The listing builds one solid part. Answer for the finished solid, in the listing's coordinates (mm). Coordinates: 2 decimals unless noted, no trailing zeros. Write each loop counter-clockwise with the first axis right and the second up, starting at its lowest first coordinate (ties: lowest second). Pieces come first, ordered by that corner, then holes.
from build123d import *

# Parameters (mm, degrees)
SKETCH_1_R          = 1.525
EXTRUDE_1_DEPTH     = 3
FILLET_1_R          = 4
CUT_EXTRUDE_1_DEPTH = 10
FILLET_2_R          = 2
SKETCH_4_R          = 2.5
CUT_EXTRUDE_2_DEPTH = 10
FILLET_3_R          = 2


with BuildPart() as part:
    # 草图1 → 凸台-拉伸1 (new body)
    with BuildSketch(Plane.XY):
        with BuildLine():
            Line((75, -15), (75, 15))
            Line((75, 15), (42.759879905, 24.346070366))
            ThreePointArc((42.759879905, 24.346070366), (42.136261187, 24.480044275), (41.5, 24.525))
            Line((41.5, 24.525), (-41.5, 24.525))
            ThreePointArc((-41.5, 24.525), (-42.136261187, 24.480044275), (-42.759879905, 24.346070366))
            Line((-42.759879905, 24.346070366), (-75, 15))
            Line((-75, 15), (-75, -15))
            Line((-75, -15), (-42.759879905, -24.346070366))
            ThreePointArc((-42.759879905, -24.346070366), (-42.136261187, -24.480044275), (-41.5, -24.525))
            Line((-41.5, -24.525), (41.5, -24.525))
            ThreePointArc((41.5, -24.525), (42.136261187, -24.480044275), (42.759879905, -24.346070366))
            Line((42.759879905, -24.346070366), (75, -15))
        make_face()
        with Locations((-71, -10)):
            Circle(SKETCH_1_R, mode=Mode.SUBTRACT)
        with Locations((71, -10)):
            Circle(SKETCH_1_R, mode=Mode.SUBTRACT)
        with Locations((-71, 10)):
            Circle(SKETCH_1_R, mode=Mode.SUBTRACT)
        with Locations((71, 10)):
            Circle(SKETCH_1_R, mode=Mode.SUBTRACT)
        with Locations((-41.5, 20)):
            Circle(SKETCH_1_R, mode=Mode.SUBTRACT)
        with Locations((-41.5, -20)):
            Circle(SKETCH_1_R, mode=Mode.SUBTRACT)
        with Locations((41.5, 20)):
            Circle(SKETCH_1_R, mode=Mode.SUBTRACT)
        with Locations((41.5, -20)):
            Circle(SKETCH_1_R, mode=Mode.SUBTRACT)
    extrude(amount=EXTRUDE_1_DEPTH)

    # 圆角1
    fillet_1_edges = [part.edges().sort_by_distance(p)[0] for p in [
        (75, 15, 1.5),
        (75, -15, 1.5),
        (-75, -15, 1.5),
        (-75, 15, 1.5),
    ]]
    fillet(fillet_1_edges, radius=FILLET_1_R)

    # 草图2 → 切除-拉伸1 (cut)
    with BuildSketch(Plane.XY.offset(3)):
        Polygon((27.82171702, 18.525), (-27.82171702, 18.525), (0, 3.413941893), align=None)
        Polygon((-38.205524372, 17.336966413), (-52, 13.338093595), (-52, -13.338093595), (-38.205524372, -17.336966413), (-6.285577396, 0), align=None)
        Polygon((27.82171702, -18.525), (0, -3.413941893), (-27.82171702, -18.525), align=None)
        Polygon((38.205524372, 17.336966413), (6.285577396, 0), (38.205524372, -17.336966413), (52, -13.338093595), (52, 13.338093595), align=None)
        Polygon((58, -14.722268277), (58, 14.722268277), (67, 12.113263316), (67, -12.113263316), align=None)
        Polygon((-67, -12.113263316), (-58, -14.722268277), (-58, 14.722268277), (-67, 12.113263316), align=None)
    extrude(amount=-CUT_EXTRUDE_1_DEPTH, mode=Mode.SUBTRACT)

    # 圆角2
    fillet_2_edges = [part.edges().sort_by_distance(p)[0] for p in [
        (-58, -14.722268277, 1.5),
        (-67, -12.113263316, 1.5),
        (-67, 12.113263316, 1.5),
        (-58, 14.722268277, 1.5),
        (0, -3.413941893, 1.5),
        (27.82171702, -18.525, 1.5),
        (-27.82171702, -18.525, 1.5),
        (-6.285577396, 0, 1.5),
        (-38.205524372, -17.336966413, 1.5),
        (-52, -13.338093595, 1.5),
        (-52, 13.338093595, 1.5),
        (-38.205524372, 17.336966413, 1.5),
        (38.205524372, 17.336966413, 1.5),
        (52, 13.338093595, 1.5),
        (52, -13.338093595, 1.5),
        (38.205524372, -17.336966413, 1.5),
        (6.285577396, 0, 1.5),
        (58, -14.722268277, 1.5),
        (58, 14.722268277, 1.5),
        (67, 12.113263316, 1.5),
        (67, -12.113263316, 1.5),
        (-27.82171702, 18.525, 1.5),
        (27.82171702, 18.525, 1.5),
        (0, 3.413941893, 1.5),
    ]]
    fillet(fillet_2_edges, radius=FILLET_2_R)

    # 草图4 → 切除-拉伸2 (cut)
    with BuildSketch(Plane(origin=(0, 0, 0), x_dir=(-1, 0, 0), z_dir=(0, 0, -1))):
        with Locations((-31.5, -14)):
            Circle(SKETCH_4_R)
    extrude(amount=-CUT_EXTRUDE_2_DEPTH, mode=Mode.SUBTRACT)

    # 圆角3
    fillet_3_edges = [part.edges().sort_by_distance(p)[0] for p in [
        (33.812155271, -14.950756542, 1.5),
        (29.443740814, -12.57810051, 1.5),
    ]]
    fillet(fillet_3_edges, radius=FILLET_3_R)


solid = part.part
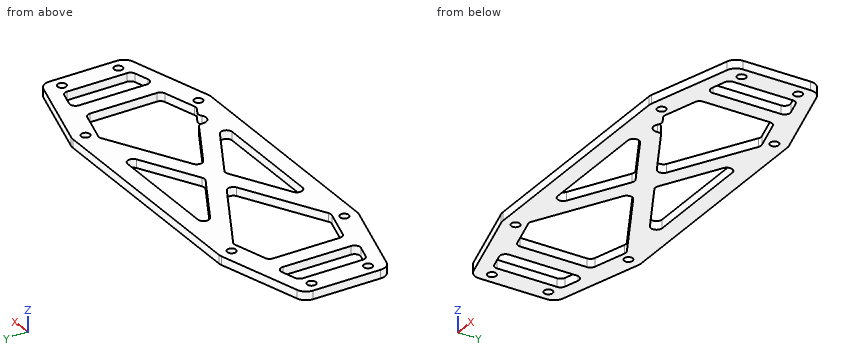
1. Section B-B on z = 1.55 is taken. State how many separate pieces and enclosed holes the cut face has, then the cut area to 3 significant figures.
Results found:
separate pieces: 1
enclosed holes: 14
area: 3,440 mm2
2. Section A-A on x = -36 is taken. Give the vertices of the cut face in (y, z) (3 decimals).
Results found:
outline: (-24.525, 0) - (-16.139, 0) - (-16.139, 3) - (-24.525, 3) - close; (16.139, 0) - (24.525, 0) - (24.525, 3) - (16.139, 3) - close
3. Find the intervals of material crossed by L1, parallel to X at y = 3, z = 1.5; L2, parallel to Y at x = -71, z = 1.1 (3 decimals); L3, parallel to Y at x = -39.5, z = 2.2 (3 decimals), in increasing order.
Results found:
L1: x = -75 to -67, -58 to -52, -11.81 to 11.81, 52 to 58, 67 to 75
L2: y = -16.16 to -11.525, -8.475 to 8.475, 11.525 to 16.16
L3: y = -24.525 to -16.962, 16.962 to 24.525
4. Section C-C on x = 54.5 is taken. Give the vertices of the cut face in (y, z), then the cut area to 3 significant figures.
Results found:
outline: (-20.94, 0) - (20.94, 0) - (20.94, 3) - (-20.94, 3) - close
area: 126 mm2
5. Flat-ended cylindrical pins translate along their axes: P1, Ø2.5, axis at x = -41.5, y = -20, coming from the -Z side; P2, Ø5, axis at x = 71, y = 10, coming from the -Z side. Find the tip coordinate at first contact, or state that the pin passes through.
Results found:
P1: passes through
P2: stops at z = 0
